Autodesk Inventor part; units mm, degrees
ref_plane "YZ Plane" through (0, 0, 0) normal (1, 0, 0) x (0, 1, 0)
ref_plane "XZ Plane" through (0, 0, 0) normal (0, 1, 0) x (-1, 0, 0)
ref_plane "XY Plane" through (0, 0, 0) normal (0, 0, 1) x (1, 0, 0)
sketch "Sketch1" plane through (0, 0, 0) normal (0, 0, 1) x (1, 0, 0)
  line L0 (-12.7, -25.4) -> (12.7, -25.4)
  line L1 (12.7, -25.4) -> (12.7, 25.4)
  line L2 (12.7, 25.4) -> (-12.7, 25.4)
  line L3 (-12.7, 25.4) -> (-12.7, -25.4)
  line L4 (-12.7, -25.4) -> (12.7, 25.4) construction
  line L5 (12.7, -25.4) -> (-12.7, 25.4) construction
  line L6 (-11.1125, 23.8125) -> (11.1125, 23.8125)
  line L7 (11.1125, 23.8125) -> (11.1125, -23.8125)
  line L8 (11.1125, -23.8125) -> (-11.1125, -23.8125)
  line L9 (-11.1125, -23.8125) -> (-11.1125, 23.8125)
  point P0 (0, 0)
  dimension "width" = 25.4
  dimension "height" = 50.8
  dimension "thickness" = 1.5875
extrude "Extrusion1" add sketch "Sketch1" along normal mid plane 165.1
sketch "Sketch5" plane through (-12.7, 25.4, 82.55) normal (0, 1, 0) x (1, 0, 0)
  point P0 (12.7, 82.55)
  point P1 (12.7, 82.55)
  point P2 (12.7, 107.95)
  point P3 (12.7, 57.15)
  dimension "d28" = 25.4
  dimension "d29" = 25.4
hole "Hole3" at (0, 25.4, 0) at (0, 25.4, -25.4) at (0, 25.4, 25.4) direction (0, -1, 0) diameter 5.1054 end through all
sketch "Sketch6" plane through (-12.7, 25.4, 82.55) normal (0, 1, 0) x (1, 0, 0)
  line L0 (12.7, 152.273) -> (12.7, 12.827) construction
  line L1 (0, 165.1) -> (25.4, 165.1) construction
  point P0 (12.7, 82.55)
  point P1 (12.7, 82.55)
  point P2 (12.7, 165.1)
  dimension "d37" = 139.446
hole "Hole4" at (0, 25.4, -69.723) at (0, 25.4, 69.723) direction (0, -1, 0) diameter 5.1054 end through all
sketch "Sketch7" plane through (12.7, -25.4, 82.55) normal (1, 0, 0) x (0, 0, -1)
  line L0 (57.9558, 25.4) -> (107.1442, 25.4) construction
  point P0 (82.55, 25.4)
  point P1 (82.55, 25.4)
  dimension "d45" = 49.1884
hole "Hole5" at (12.7, 0, 24.5942) at (12.7, 0, -24.5942) direction (-1, 0, 0) diameter 3.81 end through all
properties part number "EL2-C-001" material "Aluminum 6061"
Build history of the part. All positions in model axes, mm. A direction names the side the tool comes from. Give positions to 0.01 mm unless a question says otherwise; leave off trailing zeros. Order: outer loops, then holes, each group sorted by start corner. A loop starts at its lowest first (then second) coordinate and runs counter-clockwise, first axis right, second up. Notation, with made-up numbers: M -19.5,38.5 L 35.5,38.5 A19 ccw 35.5,63.5 Z; hole C 30,-10.5 d3. An arc over 180 degrees is marked long. Put each result on its own line as item: value.
Item 1: Slice it at C-C, the plane z = 0. Write the cut outline in (x, y), plus the area to 3 significant figures.
From the geometry:
outline: M -12.7,-25.4 L -2.55,-25.4 L -2.55,-23.81 L -11.11,-23.81 L -11.11,23.81 L -2.55,23.81 L -2.55,25.4 L -12.7,25.4 Z; M 2.55,-25.4 L 12.7,-25.4 L 12.7,25.4 L 2.55,25.4 L 2.55,23.81 L 11.11,23.81 L 11.11,-23.81 L 2.55,-23.81 Z
area: 216 mm2
Item 2: Slice it at D-D, the plane y = 0. Write the cut outline in (x, z), plus the area to 3 significant figures.
From the geometry:
outline: M -12.7,-82.55 L -11.11,-82.55 L -11.11,-26.5 L -12.7,-26.5 Z; M -12.7,-22.69 L -11.11,-22.69 L -11.11,22.69 L -12.7,22.69 Z; M -12.7,26.5 L -11.11,26.5 L -11.11,82.55 L -12.7,82.55 Z; M 11.11,-82.55 L 12.7,-82.55 L 12.7,-26.5 L 11.11,-26.5 Z; M 11.11,-22.69 L 12.7,-22.69 L 12.7,22.69 L 11.11,22.69 Z; M 11.11,26.5 L 12.7,26.5 L 12.7,82.55 L 11.11,82.55 Z
area: 500 mm2
Item 3: Two-plate mould, pull along X, no slides. Class faces 3 (the cylindrical face through (-0.112, 24.595, 67.173)), 4 (the flat face through (-11.3, 2, 82.55)), 5 (the flat face through (12.7, 0, -1)): +X half, -X half, draft (parallel to the pull), parting line (faces both ways), or undercut.
From the geometry:
face 3: undercut
face 4: draft
face 5: +X half
Item 4: Probe line 1 (Z direction, x = 11.5, y = 0); line 2 (X direction, y = -4, z = -42.5); line 3 (Z direction, x = 0, y = -24.2). List the from-to ranges inside material, lowest first. Write a range as [from, to].
From the geometry:
line 1: z = [-82.55, -26.5], [-22.69, 22.69], [26.5, 82.55]
line 2: x = [-12.7, -11.11], [11.11, 12.7]
line 3: z = [-82.55, -72.28], [-67.17, -27.95], [-22.85, -2.55], [2.55, 22.85], [27.95, 67.17], [72.28, 82.55]
Item 5: Slice it at A-A, the plane y = 16. Write the cut outline in (x, z).
From the geometry:
outline: M -12.7,-82.55 L -11.11,-82.55 L -11.11,82.55 L -12.7,82.55 Z; M 11.11,-82.55 L 12.7,-82.55 L 12.7,82.55 L 11.11,82.55 Z
Item 6: Flat gauge pin, fed straight in: pin 1 Ø3.5 at (y, z) = (0, 24.59) entering from +X. Where does the tip first touch, or does it go through?
From the geometry:
pin 1: passes through
Item 7: 3-axis set-ups, long thin cutter, end or side, ignore diameter. For faces 1 (the flat face through (3, -23.812, -1)), 2 (the cylindrical face through (-0.112, 24.595, -72.273)): which of +Z, -Z, +X, -X, +Y, -Y reach the whole face in a straight line?
From the geometry:
face 1: +Z, -Z
face 2: +Y, -Y
Item 8: Slice it at B-B, the plane x = -9.5. Write the cut outline in (y, z).
From the geometry:
outline: M -25.4,-82.55 L -23.81,-82.55 L -23.81,82.55 L -25.4,82.55 Z; M 23.81,-82.55 L 25.4,-82.55 L 25.4,82.55 L 23.81,82.55 Z
